Could you check a few things on this model? Use its own coordinates, in mm. Give positions to 0.01 mm unless a question says otherwise; leave off trailing zeros. Loops run counter-clockwise (first coordinate to the right, second up) from the corner with the lowest first, then second, coordinate; pieces in that order, holes last. Notation, with made-up numbers: M -12.5,60.25 L 36.5,60.25 A25 cw 36.5,97.25 Z; hole C 60,70 d10. An arc over 180 degrees is marked long. Use a Markdown table: item, result. Add a question column.
1) If I drill on line 1 along X through (y, z) = (25, 3.25); line 2 along Y through (x, z) = (13, 9.75), over which ranges is the centre line in solid material (lowest first)? Write a range as [from, to].
2) Suppose I cut it at C-C on z = 2. List the corners of the cut face in (x, y) for me, and give its area (3 significant figures).
3) Suppose I cut it at A-A on x = 25. List the corners of the cut face in (y, z) for me, and give its area (3 significant figures).
4) We'd pull the mould along Y, two halves only. Please class faces 1 (the flat face through (25, 0, 5)), 2 (the cylindrical face through (21.748, 10.357, 4.93)), 3 (the flat face through (36, 14, 0)): +Y half, -Y half, draft (parallel to the pull), parting line (faces both ways), or undercut.
5) Will these pins go through, and if not, where does the flat tip stop? pin 1 Ø4 at (x, y) = (38.5, 20.5) entering from +Z; pin 2 Ø18 at (x, y) = (25, 25) entering from -Z.
```python
from build123d import *

# Parameters (mm, degrees)
CYLINDER_R     = 15
CYLINDER_DEPTH = 40
BOX_W          = 50
BOX_H          = 50
BOX_DEPTH      = 10


with BuildPart() as cylinder:
    # Cylinder → Cylinder (new body)
    with BuildSketch(Plane(origin=(25, 25, -12), x_dir=(1, 0, 0), z_dir=(0, 0, 1))):
        Circle(CYLINDER_R)
    extrude(amount=CYLINDER_DEPTH)


with BuildPart() as cut:
    # Box → Box (new body)
    with BuildSketch(Plane.XY):
        with Locations((25, 25)):
            Rectangle(BOX_W, BOX_H)
    extrude(amount=BOX_DEPTH)

    # Cut: cut Cylinder
    add(cylinder.part, mode=Mode.SUBTRACT)


solid = cut.part
```
Answer block:
| question | item | result |
|---|---|---|
| 1 | line 1 | x = [0, 10], [40, 50] |
| 1 | line 2 | y = [0, 16], [34, 50] |
| 2 | outline | M 0,0 L 50,0 L 50,50 L 0,50 Z; hole C 25,25 d30 |
| 2 | area | 1,790 mm^2 |
| 3 | outline | M 0,0 L 10,0 L 10,10 L 0,10 Z; M 40,0 L 50,0 L 50,10 L 40,10 Z |
| 3 | area | 200 mm^2 |
| 4 | face 1 | -Y half |
| 4 | face 2 | undercut |
| 4 | face 3 | draft |
| 5 | pin 1 | stops at z = 10 |
| 5 | pin 2 | passes through |
